Work out the finished part from the listing and answer in its coordinate system (mm). A direction names the side the tool comes from. Coordinates: 2 decimals unless noted, no trailing zeros. Loops run counter-clockwise (first coordinate to the right, second up) from the corner with the lowest first, then second, coordinate; pieces in that order, holes last. Notation, with made-up numbers: (-38, 9) - (-17, 9) arc R17 cw to (-17, 26) - close; hole circle Ø3 at (13, -32.5). An arc over 180 degrees is marked (long way). Write each question's results on one line, items separated by ' | '. Start each with the question number.
Item 1: Each of these flat-tipped pins is pushed along its axis until it touches: pin 1 Ø4 at (x, z) = (30.5, -3) entering from +Y; pin 2 Ø14.5 at (y, z) = (0, 0) entering from +X; pin 3 Ø1 at (x, z) = (33, -27) entering from -Y. Where does it stop, or does it pass through?
Item 2: Consider probe 1 along Y at (x, z) = (16, 23.5); probe 2 along Y at (x, z) = (38, 0); probe 3 along Z at (x, y) = (37, -18). Determine where each line is inside the solid, lowest interval first. Write a range as [from, to].
Item 3: Section A-A, the plane z = 0 is taken. Write down the section's boundary in (x, y), plus the area to 3 significant figures.
Item 4: Section B-B, the plane x = 4.5 is taken. Write down the section's boundary in (y, z) (3 decimals).
Item 5: For a pull along Y with two mould halves and no side action, classify faces 1 (the face through (0, -27, -18)), 2 (the face through (20.71, -1.76, -39.96)), 3 (the face through (9.86, -31.24, 6.94)) as +Y half, -Y half, draft (parallel to the pull), parting line (faces both ways), or undercut.
Item 6: A tool of negligible diameter and unlimited length cuts with its end or side. For faces 4 (the face through (32.14, -31.24, 6.94)), 5 (the face through (0, -11, 0)), 6 (the face through (6.409, 8.923, -1.172)), from which of +Z, -Z, +X, -X, +Y, -Y can it reach the whole face along a straight path? Write none if from no direction.
from build123d import *

# Parameters (mm, degrees)
SKETCH1_R           = 40
BOSS_EXTRUDE1_DEPTH = 42
SKETCH3_R           = 32
CUT_EXTRUDE2_DEPTH  = 20
SKETCH6_R           = 30
SKETCH5_R           = 25
SKETCH2_R           = 9
CUT_EXTRUDE4_DEPTH  = 13


with BuildPart() as part:
    # Sketch1 → Boss-Extrude1 (new body)
    with BuildSketch(Plane(origin=(0, 0, 0), x_dir=(0, 0, -1), z_dir=(1, 0, 0))):
        with Locations(Location((0, 0, 0), (0, 0, 180))):
            Circle(SKETCH1_R)
    extrude(amount=BOSS_EXTRUDE1_DEPTH)

    # Sketch3 → Cut-Extrude2 (cut)
    with BuildSketch(Plane(origin=(42, 0, 0), x_dir=(0, 0, -1), z_dir=(1, 0, 0))):
        Circle(SKETCH3_R)
    cut_extrude2 = extrude(amount=-CUT_EXTRUDE2_DEPTH, mode=Mode.SUBTRACT)

    # Sketch6 → Loft1 section 0
    with BuildSketch(Plane(origin=(22, 0, 0), x_dir=(0, 0, -1), z_dir=(1, 0, 0))):
        Circle(SKETCH6_R)
    # Sketch5 → Loft1 section 1
    with BuildSketch(Plane(origin=(42, 0, 0), x_dir=(0, 0, -1), z_dir=(1, 0, 0))):
        Circle(SKETCH5_R)
    loft1 = loft()

    # Mirror5: Cut-Extrude2, Loft1 across plane
    add(cut_extrude2.mirror(Plane(origin=(21, 0, 0), x_dir=(0, 0, 1), z_dir=(1, 0, 0))), mode=Mode.SUBTRACT)
    add(loft1.mirror(Plane(origin=(21, 0, 0), x_dir=(0, 0, 1), z_dir=(1, 0, 0))))

    # Sketch2 → Cut-Extrude4 (cut)
    with BuildSketch(Plane.ZY):
        Circle(SKETCH2_R)
    cut_extrude4 = extrude(amount=-CUT_EXTRUDE4_DEPTH, mode=Mode.SUBTRACT)

    # Mirror6: Cut-Extrude4 across plane
    add(cut_extrude4.mirror(Plane(origin=(21, 0, 0), x_dir=(0, 0, 1), z_dir=(1, 0, 0))), mode=Mode.SUBTRACT)


solid = part.part
Answer key:
1) pin 1: stops at y = 39.99 | pin 2: stops at x = 29 | pin 3: stops at y = -29.96
2) probe 1: y = [-32.37, -21.72], [-16.99, 16.99], [21.72, 32.37] | probe 2: y = [-40, -32], [-26, -9], [9, 26], [32, 40] | probe 3: z = [-35.72, -26.46], [-19.11, 19.11], [26.46, 35.72]
3) outline: (0, -40) - (42, -40) - (42, -32) - (22, -32) - (22, -30) - (42, -25) - (42, -9) - (29, -9) - (29, 9) - (42, 9) - (42, 25) - (22, 30) - (22, 32) - (42, 32) - (42, 40) - (0, 40) - (0, 32) - (20, 32) - (20, 30) - (0, 25) - (0, 9) - (13, 9) - (13, -9) - (0, -9) - (0, -25) - (20, -30) - (20, -32) - (0, -32) - close | area: 2,530 mm^2
4) outline: circle Ø80 at (0, 0); circle Ø52.25 at (0, 0); hole circle Ø64 at (0, 0); hole circle Ø18 at (0, 0)
5) face 1: draft | face 2: parting line | face 3: undercut
6) face 4: +X | face 5: +Z, -Z, -X, +Y, -Y | face 6: -X
